Read the model definition and answer for the solid it produces. Units are mm, in the model's axes. Coordinates: 2 decimals unless noted, no trailing zeros. Loops run counter-clockwise (first coordinate to the right, second up) from the corner with the lowest first, then second, coordinate; pieces in that order, holes last.
Q1. Section A-A (y = -0.65) is taken. Give the vertices of the cut face in (x, z), then the cut area to 3 significant figures.
Q2. Section B-B (z = 50) is taken. Give the vertices of the cut face in (x, y), then the cut area to 3 significant figures.
Q3. Straight lines are drawn through the part: line 1 (Z direction, x = 102, y = -1.2); line 2 (Z direction, x = 37.5, y = -0.05); line 3 (Z direction, x = 85, y = 1.3). For each, find the intervals that lie inside material, in ascending order.
Q4. Section C-C (x = 33) is taken. Give the vertices of the cut face in (y, z).
Q5. Section D-D (z = 25) is taken. Give the vertices of the cut face in (x, y), then the cut area to 3 significant figures.
Q6. A flat-ended cylindrical pin translates along its axis: P1, Ø3.5, axis at x = 101.6, z = 50, coming from the -Y side. Find the tip coordinate at first contact, or state that the pin passes through.
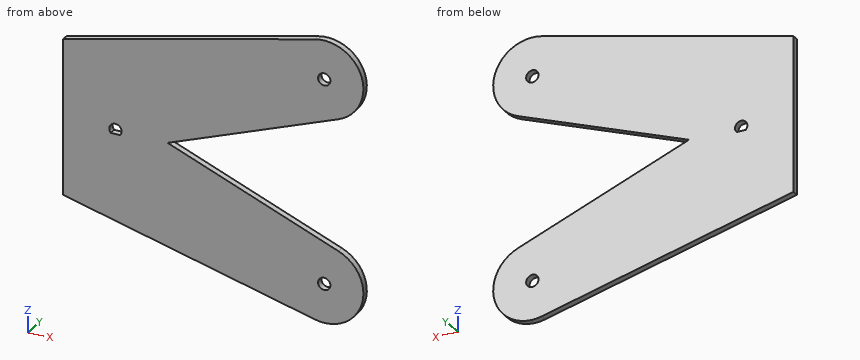
from build123d import *

# Parameters (mm, degrees)
SKETCH1_R           = 3
BOSS_EXTRUDE1_DEPTH = 1.5875


with BuildPart() as part:
    # Sketch1 → Boss-Extrude1 (new body, symmetric)
    with BuildSketch(Plane(origin=(0, 0, 0), x_dir=(1, 0, 0), z_dir=(0, 1, 0))):
        with BuildLine():
            Line((-25.4, 38.1), (97.010086235, 68.488785564))
            ThreePointArc((97.010086235, 68.488785564), (119.760857484, 55.752021858), (108.491020074, 32.240035407))
            Line((108.491020074, 32.240035407), (25.4, 0))
            Line((25.4, 0), (108.491020074, -32.240035407))
            ThreePointArc((108.491020074, -32.240035407), (119.760857484, -55.752021858), (97.010086235, -68.488785564))
            Line((97.010086235, -68.488785564), (-25.4, -38.1))
            Line((-25.4, -38.1), (-25.4, 38.1))
        make_face()
        with Locations((101.6, 50)):
            Circle(SKETCH1_R, mode=Mode.SUBTRACT)
        with Locations((101.6, -50)):
            Circle(SKETCH1_R, mode=Mode.SUBTRACT)
        with BuildLine():
            Line((-2.236067977, 2), (2.236067977, 2))
            ThreePointArc((2.236067977, 2), (0, -3), (-2.236067977, 2))
        make_face(mode=Mode.SUBTRACT)
    extrude(amount=BOSS_EXTRUDE1_DEPTH, both=True)


solid = part.part
Numbers:
1. outline: (-25.4, -38.1) - (97.01, -68.49) arc R19.05 ccw to (108.49, -32.24) - (25.4, 0) - (108.49, 32.24) arc R19.05 ccw to (97.01, 68.49) - (-25.4, 38.1) - close; hole (-2.24, -2) - (2.24, -2) arc R3 ccw (long way) to start; hole circle Ø6 at (101.6, -50); hole circle Ø6 at (101.6, 50)
1. area: 12,500 mm2
2. outline: (22.53, -1.59) - (98.6, -1.59) - (98.6, 1.59) - (22.53, 1.59) - close; (104.6, -1.59) - (120.65, -1.59) - (120.65, 1.59) - (104.6, 1.59) - close
2. area: 292 mm2
3. line 1: z = -69.05 to -52.97, -47.03 to -29.72, 29.72 to 47.03, 52.97 to 69.05
3. line 2: z = -53.72 to -4.69, 4.69 to 53.72
3. line 3: z = -65.51 to -23.13, 23.13 to 65.51
4. outline: (-1.59, -52.6) - (1.59, -52.6) - (1.59, -2.95) - (-1.59, -2.95) - close; (-1.59, 2.95) - (1.59, 2.95) - (1.59, 52.6) - (-1.59, 52.6) - close
5. outline: (-25.4, -1.59) - (89.83, -1.59) - (89.83, 1.59) - (-25.4, 1.59) - close
5. area: 366 mm2
6. P1: passes through
